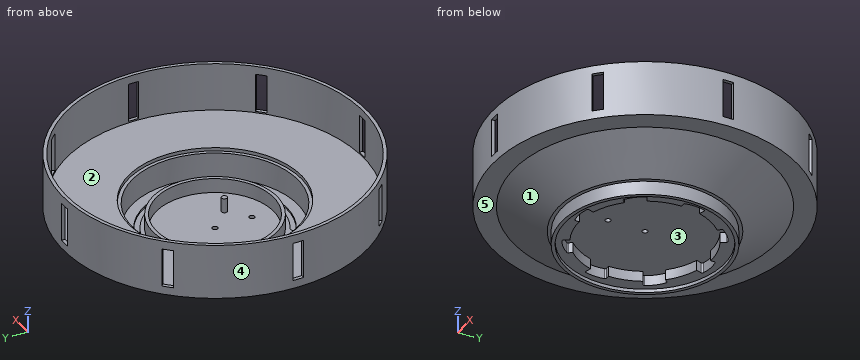
from build123d import *

# Parameters (mm, degrees)
BOSS_EXTRUDE1_DEPTH      = 1.25
BOSS_EXTRUDE1_DEPTH_BACK = 1.25
SKETCH1_R                = 60
SKETCH1_R_2              = 45
SKETCH1_R_3              = 42.5
SKETCH1_R_4              = 2
SKETCH1_3_R              = 45
SKETCH1_3_R_2            = 42.5
SKETCH1_3_R_3            = 2
BOSS_EXTRUDE2_DEPTH      = 11.75
BOSS_EXTRUDE3_DEPTH      = 20
BOSS_EXTRUDE3_DEPTH_BACK = 1.25
SKETCH1_4_R              = 62.5
SKETCH1_4_R_2            = 60
BOSS_EXTRUDE4_START      = -1.25
BOSS_EXTRUDE4_DEPTH      = 1.25
BOSS_EXTRUDE5_DEPTH      = 2.5
BOSS_EXTRUDE5_DEPTH_BACK = 2.5
SKETCH2_R                = 110
SKETCH2_R_2              = 107.5
SKETCH2_R_3              = 62.5
SKETCH3_R                = 110
SKETCH3_R_2              = 107.5
BOSS_EXTRUDE6_DEPTH      = 35
BOSS_EXTRUDE7_START      = 10
SKETCH5_R                = 60
SKETCH5_R_2              = 48
BOSS_EXTRUDE7_DEPTH      = 10
CUT_EXTRUDE1_DEPTH       = 167.287589735
FILLET1_R                = 1
CIRPATTERN2_COUNT        = 8
FILLET1_OF_CIRPATTERN2_R = 1
SKETCH7_R                = 57.5
CUT_EXTRUDE2_DEPTH       = 2.5
CUT_REVOLVE1_START       = 23.5
CUT_REVOLVE1_DEPTH       = 28
CIRPATTERN3_COUNT        = 8


# Read off the part's stored shape, not the designer's step: Cut-Revolve1
with BuildPart() as part:
    # Sketch1 → Boss-Extrude1 (new, two sides: drawn at the far end of the back side and taken through both)
    # profile 1 of 4: a face of its own
    with BuildSketch(Plane.XY.offset(-BOSS_EXTRUDE1_DEPTH_BACK)):
        Circle(SKETCH1_R)
        Circle(SKETCH1_R_2, mode=Mode.SUBTRACT)
        with BuildLine():
            ThreePointArc((-45.033320997, -26), (-42.301270189, -26.732050808), (-41.569219382, -24))
            ThreePointArc((-41.569219382, -24), (-46.364439662, 12.423314165), (-24, 41.569219382))
            ThreePointArc((-24, 41.569219382), (-23.267949192, 44.301270189), (-26, 45.033320997))
            ThreePointArc((-26, 45.033320997), (-50.228142967, 13.458590345), (-45.033320997, -26))
        make_face(mode=Mode.SUBTRACT)
        with BuildLine():
            ThreePointArc((45.033320997, -26), (44.301270189, -23.267949192), (41.569219382, -24))
            ThreePointArc((41.569219382, -24), (12.423314165, -46.364439662), (-24, -41.569219382))
            ThreePointArc((-24, -41.569219382), (-26.732050808, -42.301270189), (-26, -45.033320997))
            ThreePointArc((-26, -45.033320997), (13.458590345, -50.228142967), (45.033320997, -26))
        make_face(mode=Mode.SUBTRACT)
        with BuildLine():
            ThreePointArc((0, 52), (-2, 50), (0, 48))
            ThreePointArc((0, 48), (33.941125497, 33.941125497), (48, 0))
            ThreePointArc((48, 0), (50, -2), (52, 0))
            ThreePointArc((52, 0), (36.769552622, 36.769552622), (0, 52))
        make_face(mode=Mode.SUBTRACT)
    # profile 2 of 4: a face of its own
    with BuildSketch(Plane.XY.offset(-BOSS_EXTRUDE1_DEPTH_BACK)):
        Circle(SKETCH1_R_2)
        Circle(SKETCH1_R_3, mode=Mode.SUBTRACT)
    # profile 3 of 4: a face of its own
    with BuildSketch(Plane.XY.offset(-BOSS_EXTRUDE1_DEPTH_BACK)):
        Circle(SKETCH1_R_3)
        Circle(SKETCH1_R_4, mode=Mode.SUBTRACT)
        with Locations((14.715815051, -14.981481481)):
            Circle(SKETCH1_R_4, mode=Mode.SUBTRACT)
        with Locations((0, -27)):
            Circle(SKETCH1_R_4, mode=Mode.SUBTRACT)
    # profile 4 of 4: a face of its own
    with BuildSketch(Plane.XY.offset(-BOSS_EXTRUDE1_DEPTH_BACK)):
        with Locations((14.715815051, -14.981481481)):
            Circle(SKETCH1_R_4)
    extrude(amount=BOSS_EXTRUDE1_DEPTH + BOSS_EXTRUDE1_DEPTH_BACK)

    # Sketch1<3> → Boss-Extrude2 (add)
    # profile 1 of 2: a face of its own
    with BuildSketch(Plane.XY):
        Circle(SKETCH1_3_R)
        Circle(SKETCH1_3_R_2, mode=Mode.SUBTRACT)
    # profile 2 of 2: a face of its own
    with BuildSketch(Plane.XY):
        with Locations((14.715815051, -14.981481481)):
            Circle(SKETCH1_3_R_3)
    extrude(amount=BOSS_EXTRUDE2_DEPTH)

    # Sketch1<4> → Boss-Extrude3 (add, two sides: drawn at the far end of the back side and taken through both)
    with BuildSketch(Plane.XY.offset(-BOSS_EXTRUDE3_DEPTH_BACK)):
        Circle(SKETCH1_4_R)
        Circle(SKETCH1_4_R_2, mode=Mode.SUBTRACT)
    extrude(amount=BOSS_EXTRUDE3_DEPTH + BOSS_EXTRUDE3_DEPTH_BACK)

    # Sketch1<5> → Boss-Extrude4 (add)
    with BuildSketch(Plane.XY.offset(BOSS_EXTRUDE4_START)):
        with BuildLine():
            ThreePointArc((52, 0), (36.769552622, 36.769552622), (0, 52))
            ThreePointArc((0, 52), (-2, 50), (0, 48))
            ThreePointArc((0, 48), (33.941125497, 33.941125497), (48, 0))
            ThreePointArc((48, 0), (50, -2), (52, 0))
        make_face()
        with BuildLine():
            ThreePointArc((-26, 45.033320997), (-50.228142967, 13.458590345), (-45.033320997, -26))
            ThreePointArc((-45.033320997, -26), (-42.301270189, -26.732050808), (-41.569219382, -24))
            ThreePointArc((-41.569219382, -24), (-46.364439662, 12.423314165), (-24, 41.569219382))
            ThreePointArc((-24, 41.569219382), (-23.267949192, 44.301270189), (-26, 45.033320997))
        make_face()
        with BuildLine():
            ThreePointArc((-26, -45.033320997), (13.458590345, -50.228142967), (45.033320997, -26))
            ThreePointArc((45.033320997, -26), (44.301270189, -23.267949192), (41.569219382, -24))
            ThreePointArc((41.569219382, -24), (12.423314165, -46.364439662), (-24, -41.569219382))
            ThreePointArc((-24, -41.569219382), (-26.732050808, -42.301270189), (-26, -45.033320997))
        make_face()
    extrude(amount=BOSS_EXTRUDE4_DEPTH)

    # Sketch5 → Boss-Extrude7 (add)
    with BuildSketch(Plane(origin=(0, 0, -1.25), x_dir=(-1, 0, 0), z_dir=(0, 0, -1)).offset(BOSS_EXTRUDE7_START)):
        with Locations(Location((0, 0, 0), (0, 0, 180))):
            Circle(SKETCH5_R)
        Circle(SKETCH5_R_2, mode=Mode.SUBTRACT)
    extrude(amount=-BOSS_EXTRUDE7_DEPTH)

    # Sketch6 → Cut-Extrude1 (cut, through all)
    with BuildSketch(Plane(origin=(0, 0, -1.25), x_dir=(-1, 0, 0), z_dir=(0, 0, -1))):
        with BuildLine():
            Line((-48, 0), (-51.5, 0))
            ThreePointArc((-51.5, 0), (-52.173802074, 8.001391261), (-50.568057014, 15.868910193))
            Line((-50.568057014, 15.868910193), (-45.778413636, 14.433878376))
            ThreePointArc((-45.778413636, 14.433878376), (-47.441352502, 7.301922537), (-48, 0))
        make_face()
    cut_extrude1 = extrude(amount=CUT_EXTRUDE1_DEPTH, mode=Mode.SUBTRACT)

    # Fillet1
    fillet1_edges = [part.edges().sort_by_distance(p)[0] for p in [
        (50.568057014, 15.868910193, -6.25),
        (51.5, 0, -6.25),
    ]]
    fillet(fillet1_edges, radius=FILLET1_R)

    # CirPattern2: Cut-Extrude1 ×8 about axis
    cirpattern2_axis = Axis((0, 0, 0), (0, 0, 1))
    for i in range(1, CIRPATTERN2_COUNT):
        add(cut_extrude1.rotate(cirpattern2_axis, i * 360 / CIRPATTERN2_COUNT), mode=Mode.SUBTRACT)

    # Fillet1 of CirPattern2
    fillet1_of_cirpattern2_edges = [part.edges().sort_by_distance(p)[0] for p in [
        (24.536002018, 46.978030033, -6.25),
        (36.415999231, 36.415999231, -6.25),
        (-15.868910193, 50.568057014, -6.25),
        (0, 51.5, -6.25),
        (-46.978030033, 24.536002018, -6.25),
        (-36.415999231, 36.415999231, -6.25),
        (-50.568057014, -15.868910193, -6.25),
        (-51.5, 0, -6.25),
        (-24.536002018, -46.978030033, -6.25),
        (-36.415999231, -36.415999231, -6.25),
        (15.868910193, -50.568057014, -6.25),
        (0, -51.5, -6.25),
        (46.978030033, -24.536002018, -6.25),
        (36.415999231, -36.415999231, -6.25),
    ]]
    fillet(fillet1_of_cirpattern2_edges, radius=FILLET1_OF_CIRPATTERN2_R)

    # Sketch7 → Cut-Extrude2 (cut)
    with BuildSketch(Plane(origin=(0, 0, -11.25), x_dir=(-1, 0, 0), z_dir=(0, 0, -1))):
        Circle(SKETCH7_R)
    extrude(amount=-CUT_EXTRUDE2_DEPTH, mode=Mode.SUBTRACT)



with BuildPart() as body_2:
    # Sketch2 → Boss-Extrude5 (new, two sides: drawn at the far end of the back side and taken through both)
    # profile 1 of 2: a face of its own
    with BuildSketch(Plane.XY.offset(20).offset(-BOSS_EXTRUDE5_DEPTH_BACK)):
        Circle(SKETCH2_R)
        Circle(SKETCH2_R_2, mode=Mode.SUBTRACT)
    # profile 2 of 2: a face of its own
    with BuildSketch(Plane.XY.offset(20).offset(-BOSS_EXTRUDE5_DEPTH_BACK)):
        Circle(SKETCH2_R_2)
        Circle(SKETCH2_R_3, mode=Mode.SUBTRACT)
    extrude(amount=BOSS_EXTRUDE5_DEPTH + BOSS_EXTRUDE5_DEPTH_BACK)

    # Sketch3 → Boss-Extrude6 (add)
    with BuildSketch(Plane.XY.offset(22.5)):
        Circle(SKETCH3_R)
        Circle(SKETCH3_R_2, mode=Mode.SUBTRACT)
    extrude(amount=BOSS_EXTRUDE6_DEPTH)

    # Cut-Revolve1 outline → Cut-Revolve1 (cut)
    with BuildSketch(Plane.XY.offset(CUT_REVOLVE1_START)):
        with BuildLine():
            Line((-3.838944637, 109.932990972), (-3.751695896, 107.434513905))
            ThreePointArc((-3.751695896, 107.434513905), (0, 107.5), (3.751695896, 107.434513905))
            Line((3.751695896, 107.434513905), (3.838944637, 109.932990972))
            ThreePointArc((3.838944637, 109.932990972), (0, 110), (-3.838944637, 109.932990972))
        make_face()
    cut_revolve1 = extrude(amount=CUT_REVOLVE1_DEPTH, mode=Mode.SUBTRACT)

    # CirPattern3: Cut-Revolve1 ×8 about axis
    cirpattern3_axis = Axis((0, 0, 0), (0, 0, 1))
    for i in range(1, CIRPATTERN3_COUNT):
        add(cut_revolve1.rotate(cirpattern3_axis, i * 360 / CIRPATTERN3_COUNT), mode=Mode.SUBTRACT)


with BuildPart() as part_1:
    add(part.part)

    add(body_2.part)  # Revolve1 merges body 2
    # Sketch9 → Revolve1 (revolve)
    with BuildSketch(Plane(origin=(0, 0, 0), x_dir=(1, 0, 0), z_dir=(0, 1, 0))):
        Polygon((62.5, 1.25), (94.975952642, -17.5), (62.5, -17.5), align=None)
    revolve(axis=Axis((0, 0, 0), (0, 0, 1)))


solid = part_1.part
The model under review builds one solid part; all positions refer to its coordinate system, in mm. Face numbers are marked on the shaded views. A direction names the side the tool comes from. Give positions to 0.01 mm unless a question says otherwise; leave off trailing zeros. Write each loop counter-clockwise with the first axis right and the second up, starting at its lowest first coordinate (ties: lowest second). Pieces come first, ordered by that corner, then holes. Notation, with made-up numbers: M 53.5,84.5 L 68.5,84.5 A8 cw 68.5,90.5 Z; hole C -28.5,48.5 d3. An arc over 180 degrees is marked long. One line per question, with ' | ' between items. Start each with the question number.
Item 1: We need section A-A on z = 32. Give the number of separate pieces and of enclosed holes in the cut face, plus the area to 3 significant figures.
Item 2: We need section B-B on z = 8. Write out the cut boundary in (x, y).
Item 3: Wall thickness on line 1 (X direction, y = 80.5, z = 44) (3 decimals); line 2 (Y direction, x = -32, z = 37); line 3 (X direction, y = -35, z = -6): over which ranges is each line inside the solid? List them lowest first. Write a range as from..to.
Item 4: For pin 1 (3 mm diameter, centred on x = -44, z = 39.5, fed in from -Y); pin 2 (2 mm diameter, centred on x = 17, y = 6.5, fed in from +Z); pin 3 (6 mm diameter, centred on x = 79.5, y = 25, fed in from +Z); pin 4 (3 mm diameter, centred on x = 0, y = 0, fed in from -Z), all flat-tipped, find the tip position at first contact; note any pin that passes through.
Item 5: For the marked faces 1 and 2, list the 3-axis set-ups (+Z, -Z, +X, -X, +Y, -Y) from which the entire face can be reached by the end or side of a thin tool; tool diameter is ignored.
Item 6: Draft analysis for pull direction Y (two halves, no side actions). For the marked faces 3, 4 and 5, state which applies: released by +Y, released by -Y, zero draft, split by the parting line, or undercut.
Results found:
1) separate pieces: 8 | enclosed holes: 0 | area: 1,560 mm2
2) outline: C 0,0 d157.04; C 0,0 d90; C 14.72,-14.98 d4; hole C 0,0 d120; hole C 0,0 d85
3) line 1: x = -74.965..-71.246, 71.246..74.965 | line 2: y = -105.24..-102.63, 102.63..105.24 | line 3: x = -48.73..-35, 32.85..35, 38.47..48.73
4) pin 1: stops at y = -101.46 | pin 2: stops at z = 1.25 | pin 3: stops at z = 22.5 | pin 4: passes through
5) face 1: -Z | face 2: +Z
6) face 3: undercut | face 4: split by the parting line | face 5: zero draft
